```python
from build123d import *

# Parameters (mm, degrees)
BOSS_EXTRUDE1_DEPTH = 5
SKETCH3_W           = 47
SKETCH3_H           = 25
BOSS_EXTRUDE2_DEPTH = 8
RIB2_REACH          = 56.854
SKETCH9_WALL_W      = 137.164549338
SKETCH9_WALL_H      = 6
SKETCH2_R           = 5.5
SKETCH2_R_2         = 4.2
CUT_EXTRUDE1_DEPTH  = 5
SKETCH4_R           = 2.575
CUT_EXTRUDE2_DEPTH  = 8
SKETCH11_W          = 5.5
SKETCH11_H          = 5
BOSS_EXTRUDE5_DEPTH = 7
SKETCH12_R          = 4.941066883
BOSS_EXTRUDE6_DEPTH = 1
SKETCH7_R           = 5.5
CUT_EXTRUDE3_DEPTH  = 4
SKETCH10_W          = 11.059960659
SKETCH10_H          = 2
CUT_EXTRUDE4_DEPTH  = 4
CHAMFER1_SIZE       = 6
CHAMFER2_SIZE       = 7
CHAMFER4_SIZE       = 2
LPATTERN1_COUNT     = 2
LPATTERN1_PITCH     = 18
CHAMFER5_SIZE       = 2
CHAMFER6_SIZE       = 5


# Some blends are built 0.0001 mm under size
with BuildPart() as part:
    # Sketch1 → Boss-Extrude1 (new body)
    with BuildSketch(Plane(origin=(0, 0, 0), x_dir=(1, 0, 0), z_dir=(0, 1, 0))):
        Polygon((20, 20), (20, 12), (9, 12), (9, -20), (-27, -20), (-27, 20), align=None)
    extrude(amount=BOSS_EXTRUDE1_DEPTH)

    # Sketch3 → Boss-Extrude2 (add)
    with BuildSketch(Plane(origin=(0, 0, -20), x_dir=(-1, 0, 0), z_dir=(0, 0, -1))):
        with Locations((3.5, -7.5)):
            Rectangle(SKETCH3_W, SKETCH3_H)
    extrude(amount=-BOSS_EXTRUDE2_DEPTH)

    # Sketch9 wall → Rib2 (add, up to next)
    with BuildSketch(Plane(origin=(-27, -9, -3), x_dir=(0, 0.707106781187, 0.707106781187), z_dir=(0, 0.707106781187, -0.707106781187)), mode=Mode.PRIVATE) as rib2_sk1:
        with Locations((0, 3)):
            Rectangle(SKETCH9_WALL_W, SKETCH9_WALL_H)
    rib2_tool1 = extrude(rib2_sk1.sketch, amount=RIB2_REACH, mode=Mode.PRIVATE) - part.part
    add(rib2_tool1.solids().sort_by_distance((-27, -9, -3))[0])

    # Sketch2 → Cut-Extrude1 (cut)
    with BuildSketch(Plane(origin=(0, 5, 0), x_dir=(1, 0, 0), z_dir=(0, 1, 0))):
        with Locations(Location((-1, -10, 0), (0, 0, 270))):
            Circle(SKETCH2_R)
        with Locations(Location((-18.5, -10, 0), (0, 0, 270))):
            Circle(SKETCH2_R_2)
        Polygon((9, -5.320508076), (16.5, -0.990381057), (16.5, 7.669872981), (9, 12), (1.5, 7.669872981), (1.5, -0.990381057), align=None)
        Polygon((-10.36219397, -5.320508076), (-2.86219397, -0.990381057), (-2.86219397, 7.669872981), (-10.36219397, 12), (-17.86219397, 7.669872981), (-17.86219397, -0.990381057), align=None)
    extrude(amount=-CUT_EXTRUDE1_DEPTH, mode=Mode.SUBTRACT)

    # Sketch4 → Cut-Extrude2 (cut)
    with BuildSketch(Plane.XY.offset(-12)):
        with Locations((-10, -8)):
            Circle(SKETCH4_R)
        with Locations((10, -8)):
            Circle(SKETCH4_R)
    extrude(amount=-CUT_EXTRUDE2_DEPTH, mode=Mode.SUBTRACT)

    # Sketch11 → Boss-Extrude5 (add)
    with BuildSketch(Plane(origin=(0, 5, 0), x_dir=(1, 0, 0), z_dir=(0, 1, 0))):
        with Locations((-10, 22.5)):
            Rectangle(SKETCH11_W, SKETCH11_H)
        with Locations((10, 22.5)):
            Rectangle(SKETCH11_W, SKETCH11_H)
    boss_extrude5 = extrude(amount=-BOSS_EXTRUDE5_DEPTH)

    # Sketch12 → Boss-Extrude6 (add)
    with BuildSketch(Plane(origin=(0, 5, 0), x_dir=(1, 0, 0), z_dir=(0, 1, 0))):
        with Locations((-18.5, -10)):
            Circle(SKETCH12_R)
    extrude(amount=-BOSS_EXTRUDE6_DEPTH)

    # Sketch7 → Cut-Extrude3 (cut)
    with BuildSketch(Plane.XY.offset(-12)):
        with Locations((-10, -8)):
            Circle(SKETCH7_R)
        with Locations((10, -8)):
            Circle(SKETCH7_R)
    extrude(amount=-CUT_EXTRUDE3_DEPTH, mode=Mode.SUBTRACT)

    # Sketch10 → Cut-Extrude4 (cut)
    with BuildSketch(Plane.XZ):
        with Locations((-10.613093562, 9.96527114)):
            Rectangle(SKETCH10_W, SKETCH10_H)
    extrude(amount=-CUT_EXTRUDE4_DEPTH, mode=Mode.SUBTRACT)

    # Chamfer1
    chamfer1_edges = [part.edges().sort_by_distance(p)[0] for p in [
        (-27, -7.5, -20),
        (9, 2.5, 20),
        (-27, 2.5, 20),
    ]]
    chamfer(chamfer1_edges, length=CHAMFER1_SIZE)

    # Chamfer2
    chamfer2_edges = [part.edges().sort_by_distance(p)[0] for p in [
        (-27, -20, -13),
        (20, -20, -16),
    ]]
    chamfer(chamfer2_edges, length=CHAMFER2_SIZE)

    # Chamfer4
    # the kernel refuses this chamfer: 2 mm, written as the material it adds along each edge
    with BuildSketch(Plane(origin=(-19.666666667, -1.333333333, -10.666666667), x_dir=(-0.7071067811865462, -0.7071067811865488, 1.1932702685996668e-13), z_dir=(-0.5773502691896611, 0.5773502691895617, -0.5773502691896545))) as chamfer4_piece_1_section:
        Polygon((-1.414213562, 0.816496581), (1.414213562, 0.816496581), (0, -1.632993162), align=None)
    chamfer4_piece_1 = extrude(amount=2.540341184, mode=Mode.PRIVATE)
    chamfer4_piece_1 = split(chamfer4_piece_1, bisect_by=Plane(origin=(-21, 0, -12), z_dir=(0, -1, 0)), keep=Keep.TOP, mode=Mode.PRIVATE)
    chamfer4_piece_1 = split(chamfer4_piece_1, bisect_by=Plane(origin=(-21, 0, -12), z_dir=(1, 0, 0)), keep=Keep.TOP, mode=Mode.PRIVATE)
    chamfer4_piece_1 = split(chamfer4_piece_1, bisect_by=Plane(origin=(-21, 0, -12), z_dir=(0, 0, 1)), keep=Keep.TOP, mode=Mode.PRIVATE)
    add(chamfer4_piece_1)
    with BuildSketch(Plane(origin=(14.143365976, 0, -12), x_dir=(0, -0.9996219169112968, -0.027495876610586494), z_dir=(-1, 0, 0))) as chamfer4_piece_2_section:
        Polygon((CHAMFER4_SIZE * 0.999621916911, CHAMFER4_SIZE * 0.0274958766106), (-CHAMFER4_SIZE * 0.0274958766106, CHAMFER4_SIZE * 0.999621916911), (0, 0), align=None)
    chamfer4_piece_2 = extrude(amount=24.505559946, mode=Mode.PRIVATE)
    chamfer4_piece_2 = split(chamfer4_piece_2, bisect_by=Plane(origin=(1.470049267, -0.68923776, -7.652580917), z_dir=(-0.5000000000000001, 0, -0.8660254037844387)), keep=Keep.TOP, mode=Mode.PRIVATE)
    chamfer4_piece_2 = split(chamfer4_piece_2, bisect_by=Plane(origin=(-2.832243237, -0.68923776, -7.652580917), z_dir=(0.5000000000000001, 0, -0.8660254037844386)), keep=Keep.TOP, mode=Mode.PRIVATE)
    add(chamfer4_piece_2)
    with BuildSketch(Plane(origin=(-21, -23.143365976, -12), x_dir=(0.9996219169112965, 0, -0.027495876610597728), z_dir=(0, 1, 0))) as chamfer4_piece_3_section:
        Polygon((CHAMFER4_SIZE * 0.999621916911, -CHAMFER4_SIZE * 0.0274958766106), (-CHAMFER4_SIZE * 0.0274958766106, -CHAMFER4_SIZE * 0.999621916911), (0, 0), align=None)
    chamfer4_piece_3 = extrude(amount=23.143365976, mode=Mode.PRIVATE)
    chamfer4_piece_3 = split(chamfer4_piece_3, bisect_by=Plane(origin=(-20.326923077, -13.009615385, -7.009615385), z_dir=(0, 0.7071067811865476, -0.7071067811865476)), keep=Keep.TOP, mode=Mode.PRIVATE)
    add(chamfer4_piece_3)
    with BuildSketch(Plane(origin=(-21, 0, -17.143365976), x_dir=(0.9996219169112968, 0.02749587661058649, 0), z_dir=(0, 0, 1))) as chamfer4_piece_4_section:
        Polygon((CHAMFER4_SIZE * 0.999621916911, -CHAMFER4_SIZE * 0.0274958766106), (-CHAMFER4_SIZE * 0.0274958766106, -CHAMFER4_SIZE * 0.999621916911), (0, 0), align=None)
    chamfer4_piece_4 = extrude(amount=28.286731952, mode=Mode.PRIVATE)
    chamfer4_piece_4 = split(chamfer4_piece_4, bisect_by=Plane(origin=(-20.327046258, -4.990950262, 1.009049738), z_dir=(0, 0.7071067811865476, -0.7071067811865476)), keep=Keep.TOP, mode=Mode.PRIVATE)
    chamfer4_piece_4 = chamfer4_piece_4 - Plane(origin=(-18.5, -0.653916776, 10), x_dir=(0, 0, 1), z_dir=(0, 1, 0)) * Cylinder(4.2, 65, mode=Mode.PRIVATE)
    add(chamfer4_piece_4)
    with BuildSketch(Plane(origin=(-10.36219397, 0, -12), x_dir=(0, -0.9996219169112998, -0.027495876610477744), z_dir=(-1, 0, 0))) as chamfer4_piece_5_section:
        Polygon((CHAMFER4_SIZE * 0.999621916911, CHAMFER4_SIZE * 0.0274958766106), (-CHAMFER4_SIZE * 0.0274958766105, CHAMFER4_SIZE * 0.999621916911), (0, 0), align=None)
    chamfer4_piece_5 = extrude(amount=15.781172006, mode=Mode.PRIVATE)
    chamfer4_piece_5 = split(chamfer4_piece_5, bisect_by=Plane(origin=(-15.029121281, -0.686960661, -9.305548261), z_dir=(-0.5000000000000003, 0, -0.8660254037844387)), keep=Keep.TOP, mode=Mode.PRIVATE)
    add(chamfer4_piece_5)

    # LPattern1: Boss-Extrude5 ×2
    with Locations(*[(0, -i * LPATTERN1_PITCH, 0) for i in range(1, LPATTERN1_COUNT)]):
        add(boss_extrude5)

    # Chamfer5
    chamfer5_edges = [part.edges().sort_by_distance(p)[0] for p in [
        (-10, -2, -25),
        (10, -2, -25),
    ]]
    chamfer(chamfer5_edges, length=CHAMFER5_SIZE)

    # Chamfer6
    chamfer6_edges = [part.edges().sort_by_distance(p)[0] for p in [
        (-10, -13, -25),
        (10, -13, -25),
    ]]
    chamfer(chamfer6_edges, length=CHAMFER6_SIZE - 0.0001)  # a hair under: the kernel refuses the full size


solid = part.part
```
Here's how the part is built. I have some questions about the finished solid (model axes, mm). A direction names the side the tool comes from. Round coordinates to 2 decimals unless told otherwise and drop trailing zeros. Order: outer loops, then holes, each group sorted by start corner. A loop starts at its lowest first (then second) coordinate and runs counter-clockwise, first axis right, second up. Notation, with made-up numbers: M -4,84.5 L 20,84.5 A18 ccw 20,116.5 Z; hole C 29,53.25 d6. An arc over 180 degrees is marked long. Answer as CSV lines item,"result".
Item 1: Imagine slicing it at A-A on y = -8. List the corners of the cut face in (x, z) for me (3 decimals), and give its area (3 significant figures).
From the geometry:
outline,"M -27,-14 L -21,-20 L -12.575,-20 L -12.575,-16 L -15.5,-16 L -15.5,-12 L -19,-12 L -21,-10 L -21,-2 L -27,-2 Z; M -7.425,-20 L 7.425,-20 L 7.425,-16 L 4.5,-16 L 4.5,-12 L -4.5,-12 L -4.5,-16 L -7.425,-16 Z; M 12.575,-20 L 20,-20 L 20,-12 L 15.5,-12 L 15.5,-16 L 12.575,-16 Z"
area,"291 mm2"
Item 2: Imagine slicing it at B-B on x = -1. List the corners of the cut face in (y, z) for me.
From the geometry:
outline,"M -20,-20 L 5,-20 L 5,4.5 L 0,4.5 L 0,-10 L -2,-12 L -20,-12 Z; M 0,15.5 L 5,15.5 L 5,20 L 0,20 Z"
Item 3: Please list where these lines run through material, in increasing order: L1, parallel to Z at x = -1, y = 2.25; L2, parallel to Y at x = 10, z = -14; L3, parallel to X at y = 3.1, z = 10. Write a range as [from, to].
From the geometry:
L1,"[-20, 4.5], [15.5, 20]"
L2,"[-20, -13.5], [-2.5, 5]"
L3,"[-27, -22.7], [4.5, 9]"
Item 4: We'd pull the mould along Z, two halves only. Please class faces 4 (the flat face through (-14.16, 2.54, 3.13)), 5 (the flat face through (10, -19, -25)), 6 (the flat face through (12.4, -6.7, -16)): +Z half, -Z half, draft (parallel to the pull), parting line (faces both ways), or undercut.
From the geometry:
face 4,"undercut"
face 5,"-Z half"
face 6,"+Z half"
Item 5: Which directions (+Z, -Z, +X, -X, +Y, -Y) give clear straight access to the entire face, cutting with the end or side of a thin tool? Please do faces 1 (the flat face through (-9, 0, 8)), 2 (the cylindrical face through (-7.5, -12.9, -14)), 3 (the flat face through (-12.75, 2, -22)).
From the geometry:
face 1,"+Z, +X, -Y"
face 2,"+Z"
face 3,"-Z, -X, +Y, -Y"
Item 6: Imagine slicing it at C-C on z = 10. List the corners of the cut face in (x, y) for me, and give its area (3 significant figures).
From the geometry:
outline,"M -27,0 L -22.7,0 L -22.7,4 L -6.5,4 L -6.5,5 L -27,5 Z; M 4.5,0 L 9,0 L 9,5 L 4.5,5 Z"
area,"60.2 mm2"
Item 7: For pin 1 (9 mm diameter, centred on x = 8, y = -10.5, fed in from +Z); pin 2 (5.5 mm diameter, centred on x = -9.5, y = -7, fed in from +Z); pin 3 (2.5 mm diameter, centred on y = 2.5, z = 11, fed in from +X); pin 4 (12 mm diameter, centred on y = -11.5, z = 11, fed in from +X), each with a flat end and sliding along its axis, tell me the tip position at first contact or that it passes through.
From the geometry:
pin 1,"z = -12"
pin 2,"z = -16"
pin 3,"x = 9"
pin 4,"through"
Item 8: Imagine slicing it at D-D on x = 17. List the corners of the cut face in (y, z) for me, and give its area (3 significant figures).
From the geometry:
outline,"M -16,-20 L 5,-20 L 5,-12 L -16,-12 Z"
area,"168 mm2"
